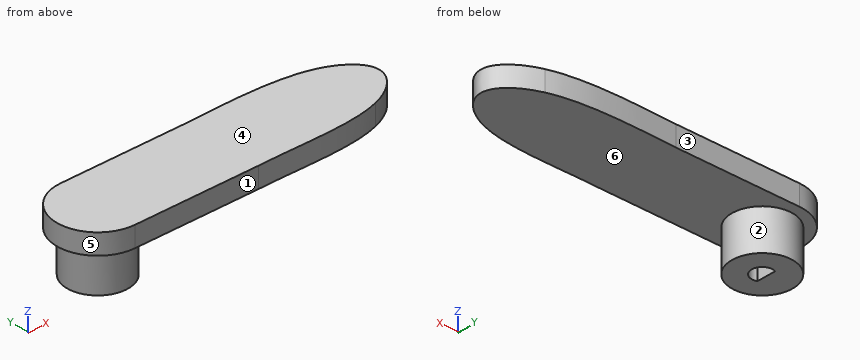
```python
from build123d import *

# Parameters (mm, degrees)
F1_R     = 9.525
F2_DEPTH = 12.7
F3_DEPTH = 6.35
F5_DEPTH = 6.35


with BuildPart() as f2:
    # F1 (on Top) → F2 (new body)
    with BuildSketch(Plane.XY):
        Circle(F1_R)
    extrude(amount=F2_DEPTH)

    # F0 (on Top) → F3 (cut)
    with BuildSketch(Plane.XY):
        with BuildLine():
            Line((-1.27, 3.048), (-1.27, -3.048))
            ThreePointArc((-1.27, -3.048), (3.302, 0), (-1.27, 3.048))
        make_face()
    extrude(amount=F3_DEPTH, mode=Mode.SUBTRACT)

    # F4 (on face) → F5 (join)
    with BuildSketch(Plane.XY.offset(12.7)):
        with BuildLine():
            add(Edge.make_bspline(
                [(78.1465370953, 10.1726271266), (84.5997905756, 7.9514466281), (93.2222153183, 0.1048863469), (84.5556786618, -8.2715012229), (78.1465370953, -10.4653070771)],
                knots=[0.309244335, 0.309244335, 0.309244335, 0.309244335, 0.4993866301, 0.6908259731, 0.6908259731, 0.6908259731, 0.6908259731], degree=3))
            Line((78.1465370953, 10.1726271266), (78.1465370953, -10.4653070771))
        make_face()
        with BuildLine():
            ThreePointArc((0, 12.7), (8.9802561211, 8.9802561211), (12.7, 0))
            ThreePointArc((12.7, 0), (8.9802561211, -8.9802561211), (0, -12.7))
            Line((0, -12.7), (39.0732685476, -12.7))
            add(Edge.make_bspline(
                [(78.1465370953, -10.4653070771), (67.795790613, -14.0082976621), (52.0691349766, -12.3123618235), (39.0732685476, -12.7)],
                knots=[0.6908259731, 0.6908259731, 0.6908259731, 0.6908259731, 1, 1, 1, 1], degree=3))
            Line((78.1465370953, -10.4653070771), (78.1465370953, 10.1726271266))
            add(Edge.make_bspline(
                [(39.0732685476, 12.7), (51.4508770451, 12.9306208488), (67.6510706324, 13.7851189498), (78.1465370953, 10.1726271266)],
                knots=[0, 0, 0, 0, 0.309244335, 0.309244335, 0.309244335, 0.309244335], degree=3))
            Line((39.0732685476, 12.7), (0, 12.7))
        make_face()
        with BuildLine():
            Line((0, 9.525), (0, 12.7))
            ThreePointArc((0, 12.7), (-12.7, 0), (0, -12.7))
            Line((0, -12.7), (0, -9.525))
            ThreePointArc((0, -9.525), (-9.525, 0), (0, 9.525))
        make_face()
        with BuildLine():
            ThreePointArc((0, -12.7), (8.9802561211, -8.9802561211), (12.7, 0))
            ThreePointArc((12.7, 0), (8.9802561211, 8.9802561211), (0, 12.7))
            Line((0, 12.7), (0, 9.525))
            ThreePointArc((0, 9.525), (6.7351920908, 6.7351920908), (9.525, 0))
            ThreePointArc((9.525, 0), (6.7351920908, -6.7351920908), (0, -9.525))
            Line((0, -9.525), (0, -12.7))
        make_face()
        with BuildLine():
            ThreePointArc((9.525, 0), (6.7351920908, 6.7351920908), (0, 9.525))
            Line((0, 9.525), (0, -9.525))
            ThreePointArc((0, -9.525), (6.7351920908, -6.7351920908), (9.525, 0))
        make_face()
        with BuildLine():
            Line((0, -9.525), (0, 9.525))
            ThreePointArc((0, 9.525), (-9.525, 0), (0, -9.525))
        make_face()
    extrude(amount=F5_DEPTH)


solid = f2.part
```
Check sheet for the modelled part. Datum: model origin and axes. Units: mm. Face numbers are marked on the shaded views. A direction names the side the tool comes from. Round coordinates to 2 decimals unless told otherwise and drop trailing zeros. Loops run counter-clockwise (first coordinate to the right, second up) from the corner with the lowest first, then second, coordinate; pieces in that order, holes last. Notation, with made-up numbers: (-12.75, -26.5) - (17.25, -26.5) arc R19 cw to (17.25, -2.5) - close; hole circle Ø7 at (-23, 43). An arc over 180 degrees is marked (long way). Write item = value, one per line. Start each with the question number.
Q1. Release check for a two-part mould opening along Z. For the marked faces 4, 5 and 6 record: pulls with the +Z half, pulls with the -Z half, needs draft (parallel to the pull), parting line crosses it, or undercut.
Q2. Thickness scan on L1, parallel to Y at x = 0, z = 2.75 (3 decimals); L2, parallel to Z at x = 54, y = -11.5; L3, parallel to Y at x = 11, z = 13.5. Record the ranges inside material, lowest first.
Q3. Section check C-C (z = 9). Record the boundary of the cut face in (x, y) (3 decimals), plus the area to 3 significant figures.
Q4. Section check A-A (z = 5). Record the boundary of the cut face in (x, y) (3 decimals), plus the area to 3 significant figures.
Q5. Depth check by flat-ended pin: P1, Ø13, axis at x = 26, y = 6.5, coming from the -Z side; P2, Ø3, axis at y = -1.5, z = 3, coming from the +X side (3 decimals); P3, Ø5, axis at x = 19, z = 15.5, coming from the +Y side; P4, Ø8, axis at x = 49.5, z = 7.5, coming from the +Y side. Enter the tip coordinate at first touch or a pass-through.
Q6. Section check B-B (x = 27). Record the boundary of the cut face in (y, z).
Q7. Access from +Z, -Z, +X, -X, +Y, -Y to the whole of each face (thin tool, end or side, straight path). Record for the marked faces 1, 2 and 3.
Derived:
q1.face_4 = pulls with the +Z half
q1.face_5 = needs draft
q1.face_6 = pulls with the -Z half
q2.L1 = -9.525 to -3.302, 3.302 to 9.525
q2.L2 = 12.7 to 19.05
q2.L3 = -12.7 to 12.7
q3.outline = circle Ø19.05 at (0, 0)
q3.area = 285 mm^2
q4.outline = circle Ø19.05 at (0, 0); hole (-1.27, -3.048) arc R3.302 ccw (long way) to (-1.27, 3.048) - close
q4.area = 260 mm^2
q5.P1 = 12.7
q5.P2 = 9.525
q5.P3 = 12.7
q5.P4 = through
q6.outline = (-12.7, 12.7) - (12.7, 12.7) - (12.7, 19.05) - (-12.7, 19.05) - close
q7.face_1 = +Z, -Z, -X, -Y
q7.face_2 = -Z
q7.face_3 = +Z, -Z, -X, +Y
